from build123d import *

# Parameters (mm, degrees)
F0_W      = 60
F0_H      = 50
F1_DEPTH  = 25
F2_W      = 57
F2_H      = 47
F3_DEPTH  = 22
F4_W      = 26
F4_H      = 16
F5_DEPTH  = 1.6986841711
F7_D      = 5.5
F7_DEPTH  = 1.6986841711
F8_D      = 5.5
F8_DEPTH  = 1.6986841711
F10_D     = 15.5
F10_DEPTH = 1.3033158289


with BuildPart() as f1:
    # F0 (on Top) → F1 (new body)
    with BuildSketch(Plane.XY):
        with Locations((6.6355607659, 0.0492307718)):
            Rectangle(F0_W, F0_H)
    extrude(amount=F1_DEPTH)

    # F2 (on face) → F3 (cut)
    with BuildSketch(Plane.XY.offset(25)):
        with Locations((6.679061912, -0.1484533993)):
            Rectangle(F2_W, F2_H)
    extrude(amount=-F3_DEPTH, mode=Mode.SUBTRACT)

    # F4 (on face) → F5 (cut, through all)
    with BuildSketch(Plane.XZ.offset(-23.3515466007)):
        with Locations((6.098437123, 12.1760265902)):
            Rectangle(F4_W, F4_H)
    extrude(amount=-F5_DEPTH, mode=Mode.SUBTRACT)

    # F7 (through all, one way)
    with BuildSketch(Plane.XZ.offset(-23.3515466007)):
        with Locations((-12.4521832913, 12.988736853)):
            Circle(F7_D / 2)
    extrude(amount=-F7_DEPTH, mode=Mode.SUBTRACT)

    # F8 (through all, one way)
    with BuildSketch(Plane.XZ.offset(-23.3515466007)):
        with Locations((24.6084798127, 12.988736853)):
            Circle(F8_D / 2)
    extrude(amount=-F8_DEPTH, mode=Mode.SUBTRACT)

    # F10 (through all, one way)
    with BuildSketch(Plane(origin=(0, -23.6484533993, 0), x_dir=(-1, 0, 0), z_dir=(0, 1, 0))):
        with Locations((-6.3858297653, 19.8415778577)):
            Circle(F10_D / 2)
    extrude(amount=-F10_DEPTH, mode=Mode.SUBTRACT)


solid = f1.part
Input: part model. Units: mm. Frame: model coordinates. A direction names the side the tool comes from. Give positions to 0.01 mm unless a question says otherwise; leave off trailing zeros. Order: outer loops, then holes, each group sorted by start corner. A loop starts at its lowest first (then second) coordinate and runs counter-clockwise, first axis right, second up. Notation, with made-up numbers: (0, -38.5) - (37, -38.5) arc R18 cw to (37, -22.5) - close; hole circle Ø11 at (-5.5, -39.5). An arc over 180 degrees is marked (long way). Answer as a JSON object with one key per item and string values. Group by question number.
Q1. Line query: probe 1 along Y at (x, z) = (7.5, 3.5); probe 2 along X at (y, z) = (0.5, 21); probe 3 along Z at (x, y) = (29.5, -2). Output: solid intervals per line, ascending.
Q2. Cut plane D-D, the plane z = 6. Output: boundary loops of the cut face in (x, y).
Q3. Cut plane A-A, the plane x = 23.5. Output: boundary loops of the cut face in (y, z).
Q4. First-contact query: pin 1 Ø4.5 at (x, z) = (24.61, 12.99) entering from +Y. Flat tip, straight axial feed; report the tip coordinate or a pass-through.
Q5. Set-up query: faces 1 (the face through (6, 23.352, 21)), 2 (the face through (-6.902, 24, 12)), 3 (the face through (6.635, -24.29, 12.096)). Return all of +Z, -Z, +X, -X, +Y, -Y with unobstructed straight access to the full face (end or side cutting, diameter ignored); none if empty.
Q6. Cut plane C-C, the plane z = 11.25. Output: boundary loops of the cut face in (x, y), then the cut area to 3 significant figures.
Q7. Mould query, pull axis X, two halves, no side actions, for faces 4 (the face through (-23.364, 0, 12)), 5 (the face through (6, 24, 25)), 6 (the face through (6.3, -23.648, 11.7)). Classes: pulls with the +X half, pulls with the -X half, needs draft (parallel to the pull), parting line crosses it, or undercut.
Q8. Cut plane B-B, the plane y = 22.5. Output: boundary loops of the cut face in (x, z), then the cut area to 3 significant figures.
Results:
{
 "1": {"probe 1": "-24.95 to -23.65, 23.35 to 25.05", "probe 2": "-23.36 to -21.82, 35.18 to 36.64", "probe 3": "0 to 3"},
 "2": {"outline": "(-23.36, -24.95) - (36.64, -24.95) - (36.64, 25.05) - (19.1, 25.05) - (19.1, 23.35) - (35.18, 23.35) - (35.18, -23.65) - (-21.82, -23.65) - (-21.82, 23.35) - (-6.9, 23.35) - (-6.9, 25.05) - (-23.36, 25.05) - close"},
 "3": {"outline": "(-24.95, 0) - (25.05, 0) - (25.05, 10.47) - (23.35, 10.47) - (23.35, 3) - (-23.65, 3) - (-23.65, 25) - (-24.95, 25) - close; (23.35, 15.51) - (25.05, 15.51) - (25.05, 25) - (23.35, 25) - close"},
 "4": {"pin 1": "y = -23.65"},
 "5": {"face 1": "+Z", "face 2": "+Y", "face 3": "-Y"},
 "6": {"outline": "(-23.36, -24.95) - (36.64, -24.95) - (36.64, 25.05) - (26.74, 25.05) - (26.74, 23.35) - (35.18, 23.35) - (35.18, -23.65) - (-21.82, -23.65) - (-21.82, 23.35) - (-14.58, 23.35) - (-14.58, 25.05) - (-23.36, 25.05) - close; (-10.32, 23.35) - (-6.9, 23.35) - (-6.9, 25.05) - (-10.32, 25.05) - close; (19.1, 23.35) - (22.48, 23.35) - (22.48, 25.05) - (19.1, 25.05) - close", "area": "262 mm^2"},
 "7": {"face 4": "pulls with the -X half", "face 5": "needs draft", "face 6": "undercut"},
 "8": {"outline": "(-23.36, 0) - (36.64, 0) - (36.64, 25) - (35.18, 25) - (35.18, 3) - (-21.82, 3) - (-21.82, 25) - (-23.36, 25) - close", "area": "246 mm^2"}
}
